```python
from build123d import *

# Parameters (mm, degrees)
F1_DEPTH  = 16
F2_W      = 70
F2_H      = 3
F3_DEPTH  = 2
F4_W      = 50
F4_H      = 14
F5_DEPTH  = 2
F6_R      = 1
F9_DEPTH  = 2
F11_DEPTH = 38.001
F13_D     = 4
F14_R     = 3
F14_R_2   = 2
F15_DEPTH = 5
F16_R     = 3


# Not quite as in the source:
# - a pattern or mirror of a feature is missing from the dataset's text; its kind, count and spacing are read off the source's solid


with BuildPart() as f1:
    # F0 (on Front) → F1 (new body)
    with BuildSketch(Plane.XZ):
        with BuildLine():
            Line((94, 9), (0, 9))
            ThreePointArc((0, 9), (-9, 0), (0, -9))
            Line((0, -9), (19, -9))
            ThreePointArc((19, -9), (20.7464347921, -9.5607448848), (21.84, -11.0333563221))
            ThreePointArc((21.84, -11.0333563221), (50.8304964021, -48.2470687705), (96.6350861079, -59.5275314258))
            ThreePointArc((96.6350861079, -59.5275314258), (103.3892729035, -60.5026852737), (108.8800565509, -64.5550005668))
            Line((108.8800565509, -64.5550005668), (110.184856953, -63))
            ThreePointArc((110.184856953, -63), (104.1026052212, -58.6336361635), (96.6997621323, -57.5125503141))
            ThreePointArc((96.6997621323, -57.5125503141), (52.0235205329, -46.636858721), (23.7333333333, -10.3889272035))
            ThreePointArc((23.7333333333, -10.3889272035), (21.9107246536, -7.9345748081), (19, -7))
            Line((19, -7), (0, -7))
            ThreePointArc((0, -7), (-7, 0), (0, 7))
            Line((0, 7), (94, 7))
            Line((94, 7), (94, 9))
        make_face()
    extrude(amount=F1_DEPTH)

    # F2 (on face) → F3 (join)
    with BuildSketch(Plane.XY.offset(9)):
        with Locations((59, -17.5)):
            Rectangle(F2_W, F2_H)
    extrude(amount=-F3_DEPTH)

    # F4 (on face) → F5 (join)
    with BuildSketch(Plane.XZ.offset(19)):
        with Locations((69, 2)):
            Rectangle(F4_W, F4_H)
    extrude(amount=-F5_DEPTH)

    # F6
    f6_edges = [f1.edges().sort_by_distance(p)[0] for p in [
        (59, -19, 9),
        (69, -17, 7),
    ]]
    fillet(f6_edges, radius=F6_R)

    # F7: F1 across plane


with BuildPart() as f1_1:
    add(f1.part)
    add(f1.part.mirror(Plane.XZ))

    # F8 (on face) → F9 (cut)
    with BuildSketch(Plane.XY.offset(9)):
        with BuildLine():
            Line((94, 11.9645609066), (44, 11.9645609066))
            ThreePointArc((44, 11.9645609066), (32.0354390934, 0), (44, -11.9645609066))
            Line((44, -11.9645609066), (94, -11.9645609066))
            Line((94, -11.9645609066), (94, 11.9645609066))
        make_face()
    extrude(amount=-F9_DEPTH, mode=Mode.SUBTRACT)

    # F10 (on face) → F11 (cut, through all)
    with BuildSketch(Plane.XZ.offset(19)):
        with BuildLine():
            ThreePointArc((50, 3), (47, 0), (50, -3))
            Line((50, -3), (70, -3))
            ThreePointArc((70, -3), (73, 0), (70, 3))
            Line((70, 3), (50, 3))
        make_face()
    extrude(amount=-F11_DEPTH, mode=Mode.SUBTRACT)

    # F13 (through all)
    with Locations(Plane.XZ.offset(19)):
        with Locations((80, 1)):
            Hole(F13_D / 2)

    # F14 (on face) → F15 (join)
    with BuildSketch(Plane(origin=(0, -17, 0), x_dir=(-1, 0, 0), z_dir=(0, 1, 0))):
        with Locations((-80, 1)):
            Circle(F14_R)
        with Locations((-80, 1)):
            Circle(F14_R_2, mode=Mode.SUBTRACT)
    f15 = extrude(amount=F15_DEPTH)

    # F15_copies: F15 across plane
    add(f15.mirror(Plane.ZX))

    # F16
    f16_edges = [f1_1.edges().sort_by_distance(p)[0] for p in [
        (94, 18, -5),
        (94, -18, -5),
        (44, -18, -5),
        (44, 18, -5),
    ]]
    fillet(f16_edges, radius=F16_R)


solid = f1_1.part
```
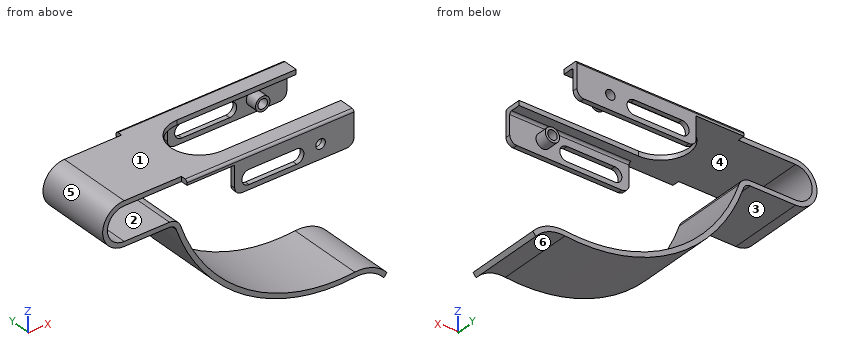
Work out the finished part from the listing and answer in its coordinate system (mm). Face numbers are marked on the shaded views. A direction names the side the tool comes from. Give positions to 0.01 mm unless a question says otherwise; leave off trailing zeros. Order: outer loops, then holes, each group sorted by start corner. A loop starts at its lowest first (then second) coordinate and runs counter-clockwise, first axis right, second up. Notation, with made-up numbers: M 12,85.25 L 40,85.25 A13 cw 40,107.25 Z; hole C 82.5,6.5 d3. An arc over 180 degrees is marked long. Return JSON: item names as keys, results as strings.
1) Each of these flat-tipped pins is pushed along its axis until it touches: pin 1 (3.5 mm diameter, centred on y = -16.5, z = 3.5, fed in from +X); pin 2 (2.5 mm diameter, centred on y = -17.5, z = 2, fed in from -X); pin 3 (12 mm diameter, centred on x = 23.5, y = 6.5, fed in from -Z). Where does it stop, or does it pass through?
Resolved:
{"pin 1": "x = 94", "pin 2": "x = 44", "pin 3": "z = -26.87"}
2) Straight lines are drawn through the part: line 1 along Z through (x, y) = (7, 0); line 2 along Y through (x, z) = (48.5, 4); line 3 along Z through (x, y) = (80, -15.9). For each, find the intervals that lie inside material, in ascending order. Write a range as [from, to].
Resolved:
{"line 1": "[-9, -7], [7, 9]", "line 2": "[-19, -17], [17, 19]", "line 3": "[-59.14, -57.12], [-2, -1], [3, 4], [7, 9]"}
3) Section C-C, the plane y = -9 is taken. Write down the section's boundary in (x, z) (3 decimals), plus the area to 3 significant figures.
Resolved:
{"outline": "M 0,-9 L 19,-9 A3 cw 21.84,-11.033 A72 ccw 96.635,-59.528 A14 cw 108.88,-64.555 L 110.185,-63 A16 ccw 96.7,-57.513 A70 cw 23.733,-10.389 A5 ccw 19,-7 L 0,-7 A7 cw 0,7 L 36.116,7 L 36.116,9 L 0,9 A9 ccw Z", "area": "389 mm^2"}
4) Section D-D, the plane z = 1 is taken. Give the number of separate pieces and of enclosed holes in the cut face, plus the area to 3 significant figures.
Resolved:
{"separate pieces": "7", "enclosed holes": "0", "area": "166 mm^2"}
5) Section A-A, the plane x = 42.5 is taken. Write down the section's boundary in (y, z), plus the area to 3 significant figures.
Resolved:
{"outline": "M -19,7 L -11.87,7 L -11.87,9 L -18,9 A1 ccw -19,8 Z; M -16,-41.94 L 16,-41.94 L 16,-39.25 L -16,-39.25 Z; M 11.87,7 L 19,7 L 19,8 A1 ccw 18,9 L 11.87,9 Z", "area": "114 mm^2"}
6) For a pull along X with two mould halves and no side action, classify the marked faces 4, 5 and 6 as +X half, -X half, draft (parallel to the pull), parting line (faces both ways), or undercut.
Resolved:
{"face 4": "draft", "face 5": "-X half", "face 6": "undercut"}
7) Section B-B, the plane x = 65.5 is taken. Write down the section's boundary in (y, z).
Resolved:
{"outline": "M -19,-5 L -17,-5 L -17,-3 L -19,-3 Z; M -19,3 L -17,3 L -17,6 A1 cw -16,7 L -11.96,7 L -11.96,9 L -18,9 A1 ccw -19,8 Z; M -16,-55.54 L 16,-55.54 L 16,-53.41 L -16,-53.41 Z; M 11.96,7 L 16,7 A1 cw 17,6 L 17,3 L 19,3 L 19,8 A1 ccw 18,9 L 11.96,9 Z; M 17,-5 L 19,-5 L 19,-3 L 17,-3 Z"}
8) A tool of negligible diameter and unlimited length cuts with its end or side. For the marked faces 1, 2 and 3, from which of +Z, -Z, +X, -X, +Y, -Y can it reach the whole face along a straight path? Write none if from no direction.
Resolved:
{"face 1": "+Z, +X, -X, +Y, -Y", "face 2": "+X, +Y, -Y", "face 3": "-Z, -X, +Y, -Y"}
